Verification items for this drawing (mm, ordinates from the low corner). A direction names the side the tool comes from. Give positions to 0.01 mm unless a question says otherwise; leave off trailing zeros. Loops run counter-clockwise (first coordinate to the right, second up) from the corner with the lowest first, then second, coordinate; pieces in that order, holes last. Notation, with made-up numbers: (25, 85) -> (82, 85) arc R21 cw to (82, 111) -> close; hole circle Ø4 at (-34, -23). An arc over 180 degrees is marked (long way). Write item = value, one per line.
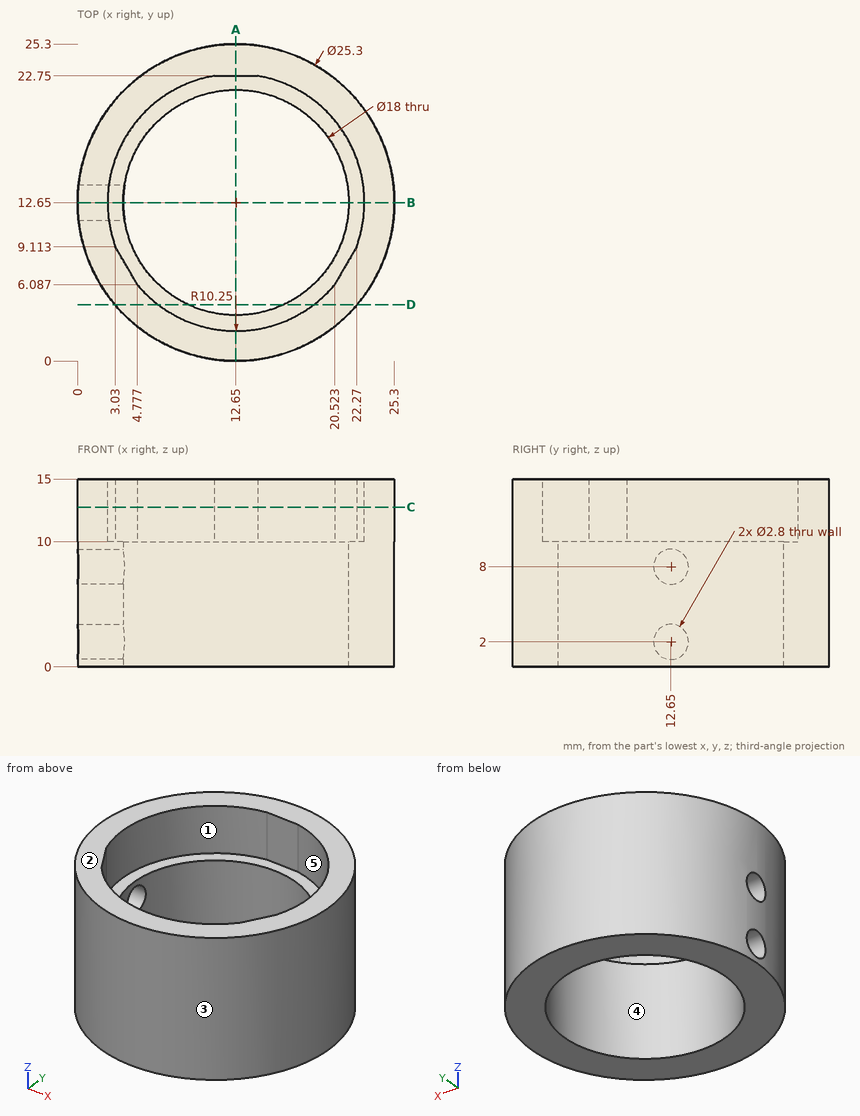
Item 1: Section check A-A, the plane x = 12.65. Record the cut outline in (y, z).
Answer:
outline = (0, 0) -> (3.65, 0) -> (3.65, 10) -> (2.4, 10) -> (2.4, 15) -> (0, 15) -> close; (21.65, 0) -> (25.3, 0) -> (25.3, 15) -> (22.75, 15) -> (22.75, 10) -> (21.65, 10) -> close
Item 2: Section check D-D, the plane y = 4.5. Record the cut outline in (x, z) (1 decimal).
Answer:
outline = (3, 0) -> (8.8, 0) -> (8.8, 10) -> (6.4, 10) -> (6.4, 15) -> (3, 15) -> close; (16.5, 0) -> (22.3, 0) -> (22.3, 15) -> (18.9, 15) -> (18.9, 10) -> (16.5, 10) -> close
Item 3: Gauge pin test, flat ends, axial feed: pin 1 (5 mm diameter, centred on y = 4.5, z = 10, fed in from +X); pin 2 (3 mm diameter, centred on y = 7, z = 8.5, fed in from -X); pin 3 (1 mm diameter, centred on y = 8.5, z = 12.5, fed in from -X). Record the tip position at first contact, or that the pin passes through.
Answer:
pin_1 = 23.97
pin_2 = 0.7
pin_3 = 0.54
Item 4: Section check C-C, the plane z = 12.75. Record the cut outline in (x, y).
Answer:
outline = circle Ø25.3 at (12.65, 12.65); hole (3.03, 9.11) -> (4.78, 6.09) arc R10.25 ccw to (20.52, 6.09) -> (22.27, 9.11) arc R10.25 ccw to (14.4, 22.75) -> (10.9, 22.75) arc R10.25 ccw to start
Item 5: Draft check along X on the marked faces 1, 2 and 3. Enter one of: +X half, -X half, draft (parallel to the pull), parting line (faces both ways), or undercut.
Answer:
face_1 = undercut
face_2 = draft
face_3 = parting line
Item 6: Thickness scan on L1, parallel to Y at x = 12.65, z = 6; L2, parallel to Y at x = 8, z = 8 (1 decimal); L3, parallel to X at y = 11.5, z = 9. Record the ranges inside material, lowest first. Write a range as [from, to].
Answer:
L1 = [0, 3.65], [21.65, 25.3]
L2 = [0.9, 4.9], [20.4, 24.4]
L3 = [0.05, 3.72], [21.58, 25.25]
Item 7: Tool access check on the marked faces 4 and 5. Record the directions out of +Z, -Z, +X, -X, +Y, -Y that give a thin tool (end or side, any length) a straight path to the whole face; none if there is none.
Answer:
face_4 = +Z, -Z
face_5 = +Z
Item 8: Section check B-B, the plane y = 12.65. Record the cut outline in (x, z).
Answer:
outline = (0, 0) -> (3.65, 0) -> (3.65, 0.6) -> (0, 0.6) -> close; (0, 3.4) -> (3.65, 3.4) -> (3.65, 6.6) -> (0, 6.6) -> close; (0, 9.4) -> (3.65, 9.4) -> (3.65, 10) -> (2.4, 10) -> (2.4, 15) -> (0, 15) -> close; (21.65, 0) -> (25.3, 0) -> (25.3, 15) -> (22.9, 15) -> (22.9, 10) -> (21.65, 10) -> close
